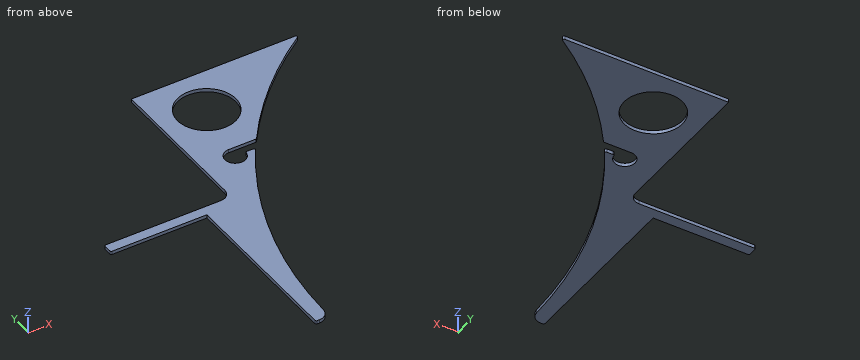
from build123d import *

# Parameters (mm, degrees)
F0_R     = 42.408979
F1_DEPTH = 2.5
F2_R     = 2
F3_R     = 15


with BuildPart() as f1:
    # F0 (on Top) → F1 (new body, symmetric)
    with BuildSketch(Plane.XY):
        with BuildLine():
            Line((5, 253), (145, 253))
            Line((145, 253), (145, 0))
            Line((145, 0), (165, 0))
            ThreePointArc((165, 0), (191.238215, 175.187092), (267.650228, 335))
            Line((267.650228, 335), (252.741245, 335))
            ThreePointArc((252.741245, 335), (227.134643, 324.393398), (237.741245, 350))
            Line((237.741245, 350), (278.1334, 350))
            ThreePointArc((278.1334, 350), (349.704058, 432.176795), (435, 500))
            Line((435, 500), (190, 500))
            Line((190, 500), (190, 268))
            Line((190, 268), (5, 268))
            Line((5, 268), (5, 253))
        make_face()
        with Locations((257.408979, 432.591021)):
            Circle(F0_R, mode=Mode.SUBTRACT)
    extrude(amount=F1_DEPTH, both=True)

    # F2
    f2_edges = [f1.edges().sort_by_distance(p)[0] for p in [
        (435, 500, 0),
        (145, 0, 0),
        (5, 268, 0),
        (5, 253, 0),
        (278.1334, 350, 0),
        (267.650228, 335, 0),
        (252.741245, 335, 0),
    ]]
    fillet(f2_edges, radius=F2_R)

    # F3
    f3_edges = [f1.edges().sort_by_distance(p)[0] for p in [
        (190, 268, 0),
        (165, 0, 0),
    ]]
    fillet(f3_edges, radius=F3_R)


solid = f1.part
Design review of the part built by this model. Coordinates are the model's own, in mm. Round coordinates to 2 decimals unless told otherwise and drop trailing zeros. Write each loop counter-clockwise with the first axis right and the second up, starting at its lowest first coordinate (ties: lowest second). Pieces come first, ordered by that corner, then holes. Notation, with made-up numbers: (43, 55.5) - (68, 55.5) arc R22 cw to (68, 74.5) - close; hole circle Ø2 at (31, 74). An arc over 180 degrees is marked (long way). Return JSON: item names as keys, results as strings. Group by question number.
Item 1: We need section C-C on z = -0.2. Write out the cut boundary in (x, y), and give its area (3 significant figures).
Item 2: We need section B-B on y = 326. Write out the cut boundary in (x, z).
Item 3: We need section A-A on x = 288.5. Write out the cut boundary in (y, z), and give its area (3 significant figures).
Item 4: For probe 1 along Y at (x, z) = (234, -1.85); probe 2 along X at (y, z) = (458.5, 0.05); probe 3 along Y at (x, z) = (296, 0.75), list the stretches that pass through material, from the lowest coordinate up. Write a range as [from, to].
Item 5: We need section D-D on x = 102. Write out the cut boundary in (y, z).
Item 6: Insertion check: P1, Ø2.5, axis at y = 67.5, z = 0, coming from the -X side; P2, Ø2.5, axis at x = 48, z = 0.5, coming from the -Y side; P3, Ø1.5, axis at y = 412, z = 1.5, coming from the +X side. Each pin has a flat end and moves straight along its axis. Give the tip position at first contact, or say it passes through.
Model answer:
{
 "1": {"outline": "(5, 255) arc R2 ccw to (7, 253) - (145, 253) - (145, 2) arc R2 ccw to (147, 0) - (150.18, 0) arc R15 ccw to (165.18, 14.63) arc R597.96 cw to (265.56, 331.89) arc R2 ccw to (263.9, 335) - (254.62, 335) arc R2 ccw to (252.64, 333.24) arc R15 cw (long way) to (237.74, 350) - (277.11, 350) arc R2 ccw to (278.73, 350.83) arc R597.96 cw to (429.49, 496.34) arc R2 ccw to (428.37, 500) - (190, 500) - (190, 283) arc R15 cw to (175, 268) - (7, 268) arc R2 ccw to (5, 266) - close; hole circle Ø84.82 at (257.41, 432.59)", "area": "34,900 mm²"},
 "2": {"outline": "(190, -2.5) - (225.74, -2.5) - (225.74, 2.5) - (190, 2.5) - close; (249.74, -2.5) - (261.68, -2.5) - (261.68, 2.5) - (249.74, 2.5) - close"},
 "3": {"outline": "(363.93, -2.5) - (403.75, -2.5) - (403.75, 2.5) - (363.93, 2.5) - close; (461.43, -2.5) - (500, -2.5) - (500, 2.5) - (461.43, 2.5) - close", "area": "392 mm²"},
 "4": {"probe 1": "y = [278.85, 320.47], [349.53, 397.23], [467.95, 500]", "probe 2": "x = [190, 223.83], [290.98, 379.12]", "probe 3": "y = [373.5, 415.01], [450.18, 500]"},
 "5": {"outline": "(253, -2.5) - (268, -2.5) - (268, 2.5) - (253, 2.5) - close"},
 "6": {"P1": "stops at x = 145", "P2": "stops at y = 253", "P3": "stops at x = 330.3"}
}
